Work out the finished part from the listing and answer in its coordinate system (mm). Face numbers are marked on the shaded views. A direction names the side the tool comes from. Coordinates: 2 decimals unless noted, no trailing zeros. Write each loop counter-clockwise with the first axis right and the second up, starting at its lowest first coordinate (ties: lowest second). Pieces come first, ordered by that corner, then holes. Notation, with made-up numbers: (63.5, 78) - (106.5, 78) arc R16 cw to (106.5, 104) - close; hole circle Ø10 at (85, -36). An arc over 180 degrees is marked (long way). One line per item, written item: value.
```python
from build123d import *

# Parameters (mm, degrees)
F0_W      = 13
F0_H      = 18.6
F1_DEPTH  = 11.7
F2_W      = 15
F2_H      = 21
F3_DEPTH  = 2
F5_START  = 1
F5_DEPTH  = 11
F6_START  = 1
F6_DEPTH  = 11
F7_R      = 1
F8_R      = 0.5
F9_W      = 5
F9_H      = 1
F10_DEPTH = 6.3
F11_SIZE  = 0.49999
F12_R     = 0.5
F13_DEPTH = 25


# Not quite as in the source:
# - a fillet or chamfer is up to 0.001 mm smaller than in the source, because OpenCascade refuses the exact size


with BuildPart() as f1:
    # F0 (on Front) → F1 (new body)
    with BuildSketch(Plane.XZ):
        with Locations((6.5, 9.3)):
            Rectangle(F0_W, F0_H)
    extrude(amount=-F1_DEPTH)

    # F2 (on Front) → F3 (join)
    with BuildSketch(Plane.XZ):
        with Locations((6.5, 9.3)):
            Rectangle(F2_W, F2_H)
    extrude(amount=F3_DEPTH)

    # F4 (on Right) → F5 (cut)
    with BuildSketch(Plane.YZ.offset(F5_START)):
        with BuildLine():
            add(Edge.make_bspline(
                [(0, 17.2755792737), (-1.1526457271, 17.1501791024), (-2.4983857291, 17.0037715611), (-3.7827872231, 16.6499606711), (-3.9660306647, 16.5956447667)],
                knots=[0, 0, 0, 0, 0.5019383156, 0.586024356, 0.586024356, 0.586024356, 0.586024356], degree=3))
            Line((0, 17.2755792737), (-3.9660306647, 17.2755792737))
            Line((-3.9660306647, 17.2755792737), (-3.9660306647, 16.5956447667))
        make_face()
        with BuildLine():
            Line((-3.9660306647, 2.481617732), (-2.1293810569, 2.481617732))
            add(Edge.make_bspline(
                [(-3.9660306647, 10.2878685019), (-3.8996200875, 10.1138282619), (-3.0167436481, 7.7059620865), (-2.5562801998, 4.9949850403), (-2.1293810569, 2.481617732)],
                knots=[0.4423976039, 0.4423976039, 0.4423976039, 0.4423976039, 0.4830426044, 1, 1, 1, 1], degree=3))
            Line((-3.9660306647, 10.2878685019), (-3.9660306647, 2.481617732))
        make_face()
        with BuildLine():
            add(Edge.make_bspline(
                [(-3.9660306647, 10.2878685019), (-3.8996200875, 10.1138282619), (-3.0167436481, 7.7059620865), (-2.5562801998, 4.9949850403), (-2.1293810569, 2.481617732)],
                knots=[0.4423976039, 0.4423976039, 0.4423976039, 0.4423976039, 0.4830426044, 1, 1, 1, 1], degree=3))
            Line((-2.1293810569, 2.481617732), (0, 2.481617732))
            Line((0, 2.481617732), (0, 17.2755792737))
            add(Edge.make_bspline(
                [(0, 17.2755792737), (-1.1526457271, 17.1501791024), (-2.4983857291, 17.0037715611), (-3.7827872231, 16.6499606711), (-3.9660306647, 16.5956447667)],
                knots=[0, 0, 0, 0, 0.5019383156, 0.586024356, 0.586024356, 0.586024356, 0.586024356], degree=3))
            Line((-3.9660306647, 16.5956447667), (-3.9660306647, 10.2878685019))
        make_face()
    extrude(amount=F5_DEPTH, mode=Mode.SUBTRACT)

    # F4 (on Right) → F6 (join)
    with BuildSketch(Plane.YZ.offset(F6_START)):
        with BuildLine():
            add(Edge.make_bspline(
                [(-3.9660306647, 10.2878685019), (-3.8996200875, 10.1138282619), (-3.0167436481, 7.7059620865), (-2.5562801998, 4.9949850403), (-2.1293810569, 2.481617732)],
                knots=[0.4423976039, 0.4423976039, 0.4423976039, 0.4423976039, 0.4830426044, 1, 1, 1, 1], degree=3))
            Line((-2.1293810569, 2.481617732), (0, 2.481617732))
            Line((0, 2.481617732), (0, 17.2755792737))
            add(Edge.make_bspline(
                [(0, 17.2755792737), (-1.1526457271, 17.1501791024), (-2.4983857291, 17.0037715611), (-3.7827872231, 16.6499606711), (-3.9660306647, 16.5956447667)],
                knots=[0, 0, 0, 0, 0.5019383156, 0.586024356, 0.586024356, 0.586024356, 0.586024356], degree=3))
            Line((-3.9660306647, 16.5956447667), (-3.9660306647, 10.2878685019))
        make_face()
        with BuildLine():
            add(Edge.make_bspline(
                [(-6.621601202, 15.6213638948), (-5.6552365252, 13.9017804778), (-4.6888718484, 12.1821970608), (-3.9660306647, 10.2878685019)],
                knots=[0, 0, 0, 0, 0.4423976039, 0.4423976039, 0.4423976039, 0.4423976039], degree=3))
            Line((-3.9660306647, 10.2878685019), (-3.9660306647, 16.5956447667))
            add(Edge.make_bspline(
                [(-3.9660306647, 16.5956447667), (-4.8681818595, 16.3282346066), (-5.7448915308, 15.9747992507), (-6.621601202, 15.6213638948)],
                knots=[0.586024356, 0.586024356, 0.586024356, 0.586024356, 1, 1, 1, 1], degree=3))
        make_face()
    extrude(amount=F6_DEPTH)

    # F7
    f7_edges = [f1.edges().sort_by_distance(p)[0] for p in [
        (14, -1, -1.2),
        (-1, -1, -1.2),
        (-1, -1, 19.8),
        (14, -1, 19.8),
        (14, -2, 9.3),
        (6.5, -2, -1.2),
        (-1, -2, 9.3),
        (6.5, -2, 19.8),
    ]]
    fillet(f7_edges, radius=F7_R)

    # F8
    f8_edges = [f1.edges().sort_by_distance(p)[0] for p in [
        (1, -4.35533, 16.47468),
        (1, -3.6216, 9.312473),
        (6.5, -6.621601, 15.621364),
        (12, -3.6216, 9.312473),
        (12, -4.35533, 16.47468),
    ]]
    fillet(f8_edges, radius=F8_R)

    # F9 (on face) → F10 (join)
    with BuildSketch(Plane(origin=(0, 11.7, 0), x_dir=(-1, 0, 0), z_dir=(0, 1, 0))):
        with Locations((-6.5, 9.3)):
            Rectangle(F9_W, F9_H)
        with Locations((-6.5, 16.3)):
            Rectangle(F9_W, F9_H)
    extrude(amount=F10_DEPTH)

    # F11 (size 0.5 in the source; OpenCascade refuses exactly that, so slightly less here)
    f11_edges = [f1.edges().sort_by_distance(p)[0] for p in [
        (4, 18, 16.3),
        (9, 18, 16.3),
        (4, 18, 9.3),
        (9, 18, 9.3),
        (6.5, 18, 16.8),
        (6.5, 18, 15.8),
        (6.5, 18, 9.8),
        (6.5, 18, 8.8),
    ]]
    chamfer(f11_edges, length=F11_SIZE)

    # F12 (on face) → F13 (cut)
    with BuildSketch(Plane.XY.offset(16.8)):
        with Locations((6.5, 16)):
            Circle(F12_R)
    extrude(amount=-F13_DEPTH, mode=Mode.SUBTRACT)


solid = f1.part
```
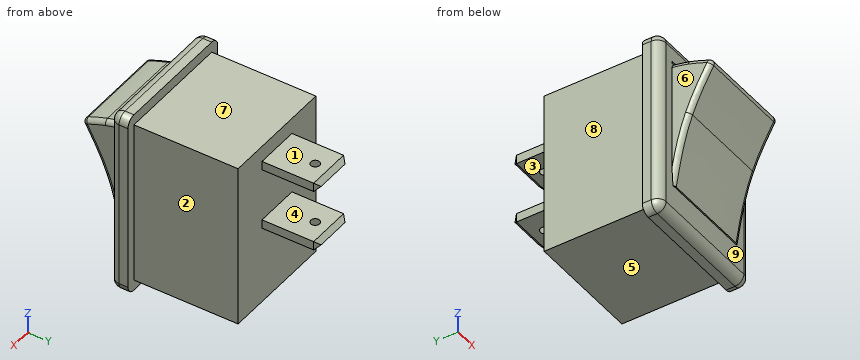
Item 1: Which of the six approach directions +Z, -Z, +X, -X, +Y, -Y give full straight-line access (tool end or side, diameter ignored) to the marked faces 5, 6, 7, 8 and 9?
Evaluation:
face 5: -Z, +X, -X, +Y
face 6: +Z, -Z, -X, -Y
face 7: +Z, +X, -X, +Y
face 8: +Z, -Z, -X, +Y
face 9: -Y
Item 2: Section C-C, the plane z = 0.75 is taken. Determine the outline of the cut face in (x, y), then the cut area to 3 significant figures.
Evaluation:
outline: (-1, -1) arc R1 ccw to (0, -2) - (13, -2) arc R1 ccw to (14, -1) - (14, 0) - (13, 0) - (13, 11.7) - (0, 11.7) - (0, 0) - (-1, 0) - close
area: 182 mm2
Item 3: Consider probe 1 along Z at (x, y) = (7.25, 13); probe 2 along Z at (x, y) = (7.5, 1.75); probe 3 along X at (y, z) = (0.25, 12.5). Determine where each line is inside the solid, lowest interval first.
Evaluation:
probe 1: z = 8.8 to 9.8, 15.8 to 16.8
probe 2: z = 0 to 18.6
probe 3: x = 0 to 13
Item 4: Given pin 1 (0.5 mm diameter, centred on y = 15, z = 16.5, fed in from +X); pin 2 (3.5 mm diameter, centred on x = 5, y = 8.5, fed in from -Z); pin 3 (5 mm diameter, centred on x = 6, y = -2, fed in from +Z); pin 4 (2 mm diameter, centred on x = 2, z = 11.5, fed in from -Y), each flat-ended and moving along its own axis, determine where each tip first touches the part or whether it passes through.
Evaluation:
pin 1: stops at x = 9
pin 2: stops at z = 0
pin 3: stops at z = 19.8
pin 4: stops at y = -4.94
Item 5: Determine the mould class of the marked faces 1, 2, 3 and 4 for opening direction Z: +Z half, -Z half, draft (parallel to the pull), parting line (faces both ways), or undercut.
Evaluation:
face 1: +Z half
face 2: draft
face 3: undercut
face 4: undercut
Item 6: Section A-A, the plane y = 16 is taken. Determine the outline of the cut face in (x, z).
Evaluation:
outline: (4, 8.8) - (6, 8.8) - (6, 9.8) - (4, 9.8) - close; (4, 15.8) - (6, 15.8) - (6, 16.8) - (4, 16.8) - close; (7, 8.8) - (9, 8.8) - (9, 9.8) - (7, 9.8) - close; (7, 15.8) - (9, 15.8) - (9, 16.8) - (7, 16.8) - close
Item 7: Section D-D, the plane x = 0.5 is taken. Determine the outline of the cut face in (y, z).
Evaluation:
outline: (-2, -0.2) arc R1 ccw to (-1, -1.2) - (0, -1.2) - (0, 0) - (11.7, 0) - (11.7, 18.6) - (0, 18.6) - (0, 19.8) - (-1, 19.8) arc R1 ccw to (-2, 18.8) - close
Item 8: Section B-B, the plane y = 13.5 is taken. Determine the outline of the cut face in (x, z), then the cut area to 3 significant figures.
Evaluation:
outline: (4, 8.8) - (9, 8.8) - (9, 9.8) - (4, 9.8) - close; (4, 15.8) - (9, 15.8) - (9, 16.8) - (4, 16.8) - close
area: 10.0 mm2
